Here's how the part is built. I have some questions about the finished solid (model axes, mm). A direction names the side the tool comes from. Give positions to 0.01 mm unless a question says otherwise; leave off trailing zeros. Loops run counter-clockwise (first coordinate to the right, second up) from the corner with the lowest first, then second, coordinate; pieces in that order, holes last.
Q1. We'd pull the mould along Z, two halves only. Please class faces 5 (the face through (30, -2, 52.5)), 6 (the face through (-30, -8.721, 39)), 7 (the face through (-30, -3.641, 4)): +Z half, -Z half, draft (parallel to the pull), parting line (faces both ways), or undercut.
Q2. For faces 1 (the face through (0, 0.388, 73)), 2 (the face through (-5.94, 3, 30)), 3 (the face through (30, -1, 63.66)), 4 (the face through (-30, -3.641, 72)), which set-ups out of +Z, -Z, +X, -X, +Y, -Y let a thin tool reach every point of the face, with its end or its side?
Q3. If we section it at B-B (z = 10.16): Please give me the cut outline in (x, y), plus the area to 3 significant figures.
Q4. If we section it at D-D (z = 72.39): Please give me the cut outline in (x, y), plus the area to 3 significant figures.
Q5. Will these pins go through, and if not, where does the flat tip stop? P1, Ø19, axis at x = -11.5, z = 55, coming from the -Y side; P2, Ø5, axis at x = 20.5, z = 60.5, coming from the -Y side.
Q6. If we section it at A-A (y = -7.75): Please give me the cut outline in (x, z).
Q7. If we section it at C-C (y = 3.75): Please give me the cut outline in (x, z), plus the area to 3 significant figures.
Q8. I need wall thicknesses on line 1 (X direction, y = -4.85, z = 72.39); line 2 (Z direction, x = -21.75, y = 4.3); line 3 (X direction, y = -6.25, z = 16.5). Which ranges of each line are inside material? Lowest first, please.
Autodesk Inventor part; units mm, degrees
ref_plane "YZ Plane" through (0, 0, 0) normal (1, 0, 0) x (0, 1, 0)
ref_plane "XZ Plane" through (0, 0, 0) normal (0, 1, 0) x (-1, 0, 0)
ref_plane "XY Plane" through (0, 0, 0) normal (0, 0, 1) x (1, 0, 0)
sketch "Sketch1" plane through (0, 0, 0) normal (0, 0, 1) x (1, 0, 0)
  line L0 (-31.75, 5.08) -> (31.75, 5.08)
  line L1 (31.75, 5.08) -> (31.75, -5.08)
  line L2 (31.75, -5.08) -> (-31.75, -5.08)
  line L3 (-31.75, -5.08) -> (-31.75, 5.08)
  point P0 (0, 0)
  dimension "d0" = 63.5
  dimension "d3" = 31.75
  dimension "d4" = 10.16
  dimension "d17" = 5.08
extrude "Extrusion1" add sketch "Sketch1" along normal blind 76.2
sketch "Sketch3" plane through (0, 0, 76.2) normal (0, 0, 1) x (1, 0, 0)
  line L0 (-27.25, 0.3875) -> (27.25, 0.3875)
  line L1 (27.25, 0.3875) -> (27.25, -0.3745)
  line L2 (27.25, -0.3745) -> (-27.25, -0.3745)
  line L3 (-27.25, -0.3745) -> (-27.25, 0.3875)
  line L4 (-31.75, 5.08) -> (-31.75, -5.08)
  point P0 (0, 0)
  point P1 (-27.25, 0.0065)
  dimension "d131" = 7.62
  dimension "d6" = 0.762
  dimension "d7" = 54.5
  dimension "d8" = 4.5
extrude "Extrusion2" cut sketch "Sketch3" against normal blind 85.1
sketch "Sketch8" plane through (0, 0, 76.2) normal (0, 0, 1) x (1, 0, 0)
  line L0 (-31.75, -5.08) -> (31.75, -5.08)
  line L1 (31.75, -5.08) -> (31.75, 5.08)
  line L2 (-31.75, -5.08) -> (31.75, -5.08)
  line L3 (31.75, -5.08) -> (31.75, 0.3875)
  line L4 (31.75, 0.3875) -> (-31.75, 0.3875)
  line L5 (27.25, 0.3875) -> (27.25, -0.3745)
  line L6 (27.25, -0.3745) -> (-27.25, -0.3745)
  line L7 (-27.25, -0.3745) -> (-27.25, 0.3875)
  line L8 (-27.25, 0.3875) -> (27.25, 0.3875)
  line L9 (-31.75, -5.08) -> (31.75, -5.08)
  line L10 (31.75, -5.08) -> (31.75, 5.08)
  line L11 (31.75, 5.08) -> (-31.75, 5.08)
  line L12 (-31.75, 5.08) -> (-31.75, -5.08)
  line L13 (-27.25, 0.3875) -> (-27.25, -0.3745)
  line L14 (-27.25, 0.3875) -> (27.25, 0.3875)
  line L15 (27.25, 0.3875) -> (27.25, -5.08)
  line L16 (27.25, -5.08) -> (-27.25, -5.08)
  line L17 (-27.25, -5.08) -> (-27.25, 0.3875)
  point P0 (0, 0)
  dimension "d30" = 0
sketch "Sketch9" plane through (-31.75, 5.08, 0) normal (0, 1, 0) x (1, 0, 0)
  line L0 (28.35, -18.7333) -> (35.15, -18.7333)
  line L1 (35.15, -18.7333) -> (35.15, -39.7333)
  line L2 (35.15, -39.7333) -> (28.35, -39.7333)
  line L3 (28.35, -39.7333) -> (28.35, -18.7333)
  line L4 (0, 0) -> (0, -76.2)
  line L5 (63.5, 0) -> (0, 0)
  point P0 (31.75, 0)
  point P1 (0, -38.1)
  dimension "d31" = 21
  dimension "d32" = 6.8
  dimension "d33" = 28.35
  dimension "d34" = 18.7333
extrude "Extrusion6" cut sketch "Sketch8" against normal blind 76.2 contours L17 L6 L15 L0
sketch "Sketch11" plane through (0, 0, 76.2) normal (0, 0, 1) x (1, 0, 0)
  point P0 (0, 0)
sketch "Sketch12" plane through (-31.75, -5.08, 0) normal (0, -1, 0) x (1, 0, 0)
  line L0 (4.5, 0) -> (4.5, 76.2)
  line L1 (0, 76.2) -> (4.5, 76.2)
  line L2 (0, 0) -> (0, 76.2)
  line L3 (0, 0) -> (4.5, 0)
  line L4 (59, 76.2) -> (59, 0)
  line L5 (59, 0) -> (63.5, 0)
  line L6 (63.5, 0) -> (63.5, 76.2)
  line L7 (59, 76.2) -> (63.5, 76.2)
  point P0 (31.75, 0)
extrude "Extrusion7" add sketch "Sketch12" along normal blind 3.641
extrude "Extrusion8" cut sketch "Sketch9" against normal blind 19.5
sketch "Sketch13" plane through (-31.75, -8.721, 0) normal (0, -1, 0) x (1, 0, 0)
  point P0 (31.75, 0)
sketch "Sketch14" plane through (27.25, 0.3875, 0) normal (-1, 0, 0) x (0, 0, 1)
  circle A0 centre (10.16, -3.3935) radius 2.55
  line L0 (76.2, 0) -> (0, 0)
  line L1 (76.2, -9.1085) -> (0, -9.1085)
  line L2 (0, -9.1085) -> (0, 0)
  point P0 (0, -0.3875)
  dimension "d41" = 5.1
  dimension "d43" = 5.715
  dimension "d44" = 10.16
extrude "Extrusion9" cut sketch "Sketch14" against normal blind 25.4
sketch "Sketch17" plane through (-31.75, -8.721, 0) normal (0, -1, 0) x (1, 0, 0)
  circle A0 centre (61.25, 3.81) radius 1.05
  line L0 (59, 0) -> (63.5, 0)
  line L1 (59, 76.2) -> (59, 0)
  circle A1 centre (2.25, 3.81) radius 1.05
  line L2 (0, 76.2) -> (0, 0)
  line L3 (0, 0) -> (4.5, 0)
  circle A2 centre (2.25, 72.39) radius 1.05
  circle A3 centre (61.25, 72.39) radius 1.05
  line L4 (4.5, 76.2) -> (0, 76.2)
  line L5 (63.5, 76.2) -> (59, 76.2)
  point P0 (31.75, 0)
  dimension "d98" = 2.1
  dimension "d99" = 3.81
  dimension "d100" = 2.25
  dimension "d101" = 2.25
  dimension "d102" = 2.1
  dimension "d103" = 3.81
  dimension "d104" = 2.1
  dimension "d105" = 2.1
  dimension "d106" = 3.81
  dimension "d107" = 3.81
  dimension "d108" = 2.25
extrude "Extrusion11" cut sketch "Sketch17" against normal blind 5.08
sketch "Sketch20" plane through (-31.75, 5.08, 0) normal (0, 1, 0) x (1, 0, 0)
  line L0 (22.81, -23.9233) -> (25.81, -23.9233)
  line L1 (25.81, -23.9233) -> (25.81, -35.9233)
  line L2 (25.81, -35.9233) -> (22.81, -35.9233)
  line L3 (22.81, -35.9233) -> (22.81, -23.9233)
  line L4 (28.35, -39.7333) -> (28.35, -18.7333)
  line L5 (35.15, -39.7333) -> (28.35, -39.7333)
  point P0 (31.75, 0)
  point P1 (31.75, -39.7333)
  dimension "d141" = 3
  dimension "d142" = 2.54
  dimension "d143" = 12
  dimension "d144" = 3.81
extrude "Extrusion14" cut sketch "Sketch20" against normal blind 25.4
sketch "Sketch18" plane through (-27.25, 0.3875, 76.2) normal (0, -1, 0) x (1, 0, 0)
  circle A0 centre (5.5, -23.82) radius 1.15
  circle A1 centre (5.5, -12.42) radius 1.05
  circle A2 centre (5.5, -12.42) radius 1.15
  line L0 (3.5, -28.62) -> (3.5, -7.62)
  circle A3 centre (5.5, -23.82) radius 1.05
  line L1 (54.5, -28.62) -> (3.5, -28.62)
  line L2 (3.5, -7.62) -> (54.5, -7.62)
  circle A4 centre (52.5, -12.42) radius 1.05
  circle A5 centre (52.5, -12.42) radius 1.15
  line L3 (54.5, -7.62) -> (54.5, -28.62)
  circle A6 centre (52.5, -23.82) radius 1.05
  circle A7 centre (52.5, -23.82) radius 1.15
  line L4 (0, 0) -> (54.5, 0)
  line L5 (54.5, 0) -> (54.5, -76.2)
  point P0 (27.25, -76.2)
  dimension "d111" = 21
  dimension "d112" = 51
  dimension "d113" = 2.1
  dimension "d114" = 2.1
  dimension "d115" = 2.1
  dimension "d116" = 2.1
  dimension "d117" = 2
  dimension "d118" = 2
  dimension "d119" = 2
  dimension "d120" = 2
  dimension "d121" = 11.4
  dimension "d122" = 4.8
  dimension "d123" = 11.4
  dimension "d124" = 4.8
  dimension "d125" = 0.1
  dimension "d126" = 0.1
  dimension "d127" = 0.1
  dimension "d128" = 0.1
  dimension "d131" = 7.62
  dimension "d132" = 0
extrude "Extrusion12" cut sketch "Sketch18" against normal blind 25.4 contours A0 | A1 | A2 | A3 | A4 | A5 | A6 | A7
sketch "Sketch21" plane through (-31.75, -8.721, 0) normal (0, -1, 0) x (1, 0, 0)
  line L0 (59, 76.2) -> (59, 0)
  line L1 (59, 69.5452) -> (61.2521, 69.5452)
  line L2 (61.2521, 69.5452) -> (61.2521, 46.6852)
  line L3 (61.2521, 46.6852) -> (59, 46.6852)
  line L4 (59, 46.6852) -> (59, 69.5452)
  line L5 (63.5, 0) -> (63.5, 76.2)
  line L6 (63.5, 76.2) -> (59, 76.2)
  point P0 (31.75, 0)
  dimension "d147" = 4.5
  dimension "d148" = 2.2479
  dimension "d149" = 6.6548
  dimension "d150" = 22.86
sketch "Sketch22" plane through (31.75, 5.08, 76.2) normal (1, 0, 0) x (0, 0, -1)
  line L0 (13.57, -4.6925) -> (13.57, 0)
  line L1 (13.57, -4.6925) -> (13.57, 0)
  line L2 (24.97, -4.6925) -> (24.97, 0)
  line L3 (22.67, -4.6925) -> (22.67, 0)
  line L4 (11.27, -4.6925) -> (11.27, 0)
  line L5 (23.7, -2.1525) -> (12.54, -2.1525)
  line L6 (12.54, -2.1525) -> (12.54, -11.0425)
  line L7 (12.54, -11.0425) -> (23.7, -11.0425)
  line L8 (23.7, -11.0425) -> (23.7, -2.1525)
  point P0 (76.2, -5.08)
  point P1 (24.97, -2.1525)
  point P2 (11.27, -2.6605)
  dimension "d152" = 8.89
  dimension "d153" = 2.54
  dimension "d169" = 1.27
  dimension "d170" = 1.27
extrude "Extrusion15" cut sketch "Sketch22" against normal blind 4.5212
sketch "Sketch24" plane through (31.75, 5.08, 76.2) normal (1, 0, 0) x (0, 0, -1)
  line L0 (37.6849, -4.6925) -> (33.6849, -4.6925)
  line L1 (33.6849, -4.6925) -> (33.6849, -7.6925)
  line L2 (33.6849, -7.6925) -> (37.6849, -7.6925)
  line L3 (37.6849, -7.6925) -> (37.6849, -4.6925)
  line L4 (0, -4.6925) -> (76.2, -4.6925)
  point P0 (76.2, -5.08)
  point P1 (23.7, -4.6925)
  dimension "d163" = 4
  dimension "d164" = 3
  dimension "d165" = 0
extrude "Extrusion16" cut sketch "Sketch24" against normal blind 9.1211
sketch "Sketch27" plane through (-27.25, 0.3875, 76.2) normal (0, -1, 0) x (1, 0, 0)
  line L0 (54.5, 0) -> (54.5, -76.2)
  line L1 (0, 0) -> (0, -76.2)
  line L2 (54.5, -29.89) -> (0, -29.89)
  line L3 (0, -29.89) -> (0, -6.35)
  line L4 (0, -6.35) -> (54.5, -6.35)
  line L5 (54.5, -6.35) -> (54.5, -29.89)
  line L6 (54.5, -28.62) -> (3.5, -28.62)
  line L7 (3.5, -7.62) -> (54.5, -7.62)
  point P0 (27.25, -76.2)
  point P1 (54.5, -6.35)
  point P2 (0, -29.89)
  dimension "d171" = 1.27
  dimension "d172" = 1.27
extrude "Extrusion17" cut sketch "Sketch27" against normal blind 1.5
properties part number "Scanner_Test_Top"
Check sheet entries:
1. face 5: undercut
1. face 6: draft
1. face 7: undercut
2. face 1: +Z, -Z, -Y
2. face 2: +Y, -Y
2. face 3: +X
2. face 4: -Y
3. outline: (-31.75, -8.72) - (-27.25, -8.72) - (-27.25, 0.39) - (27.25, 0.39) - (27.25, -0.46) - (31.75, -0.46) - (31.75, 5.08) - (-31.75, 5.08) - close; (27.25, -8.72) - (31.75, -8.72) - (31.75, -5.56) - (27.25, -5.56) - close
3. area: 357 mm2
4. outline: (-31.75, -8.72) - (-30.55, -8.72) - (-30.55, -3.64) - (-28.45, -3.64) - (-28.45, -8.72) - (-27.25, -8.72) - (-27.25, 0.39) - (27.25, 0.39) - (27.25, -8.72) - (28.45, -8.72) - (28.45, -3.64) - (30.55, -3.64) - (30.55, -8.72) - (31.75, -8.72) - (31.75, 5.08) - (-31.75, 5.08) - close
4. area: 359 mm2
5. P1: stops at y = 0.39
5. P2: stops at y = 1.89
6. outline: (-31.75, 0) - (-27.25, 0) - (-27.25, 76.2) - (-31.75, 76.2) - close; (27.25, 0) - (31.75, 0) - (31.75, 76.2) - (27.25, 76.2) - close; hole circle Ø2.1 at (-29.5, 3.81); hole circle Ø2.1 at (-29.5, 72.39); hole circle Ø2.1 at (29.5, 3.81); hole circle Ø2.1 at (29.5, 72.39)
7. outline: (-31.75, 0) - (31.75, 0) - (31.75, 76.2) - (-31.75, 76.2) - close; hole circle Ø2.3 at (-21.75, 52.38); hole circle Ø2.3 at (-21.75, 63.78); hole (-8.94, 23.92) - (-5.94, 23.92) - (-5.94, 35.92) - (-8.94, 35.92) - close; hole (-3.4, 18.73) - (3.4, 18.73) - (3.4, 39.73) - (-3.4, 39.73) - close; hole circle Ø2.3 at (25.25, 52.38); hole circle Ø2.3 at (25.25, 63.78)
7. area: 4,640 mm2
8. line 1: x = -31.75 to -30.55, -28.45 to -27.25, 27.25 to 28.45, 30.55 to 31.75
8. line 2: z = 0 to 51.23, 53.53 to 62.63, 64.93 to 76.2
8. line 3: x = -31.75 to -27.25, 27.25 to 31.75
